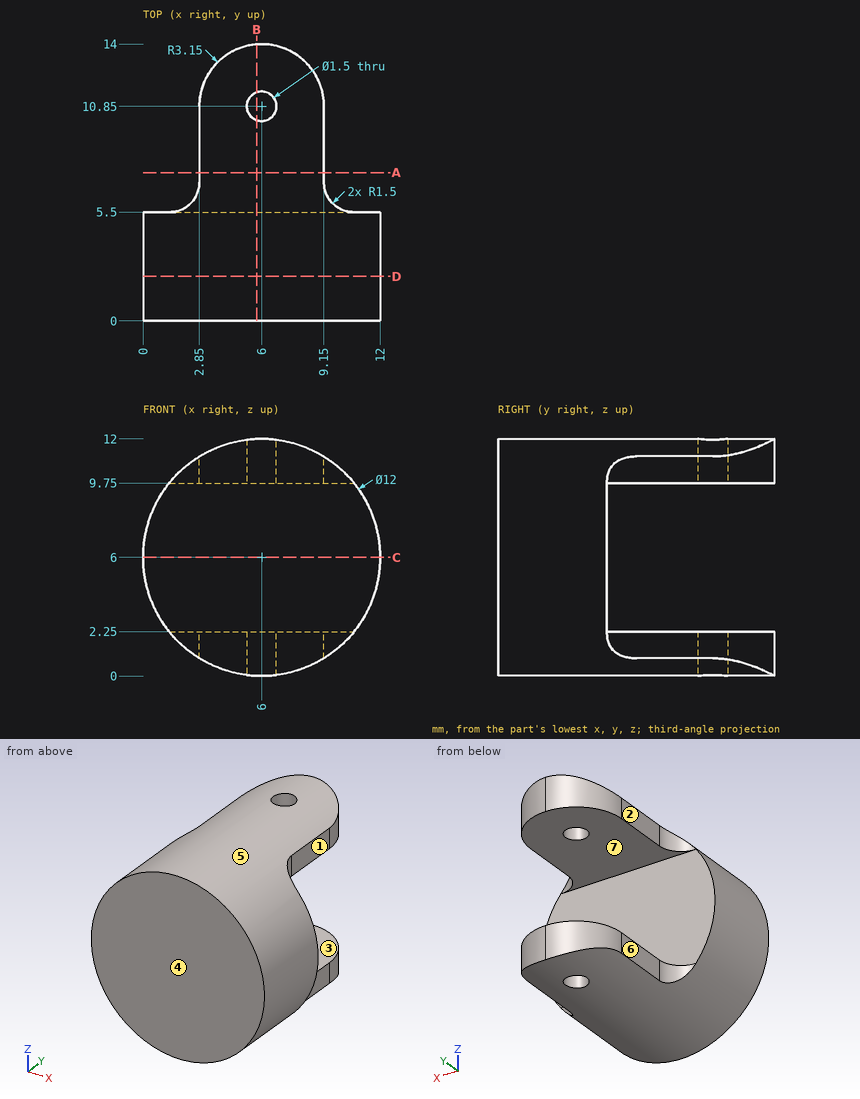
Design review of the part shown in the three views and the two pictorial views. Dimensions are in mm from the part's minimum x, y and z. A direction names the side the tool comes from. Round coordinates to 2 decimals unless told otherwise and drop trailing zeros. Loops run counter-clockwise (first coordinate to the right, second up) from the corner with the lowest first, then second, coordinate; pieces in that order, holes last. Notation, with made-up numbers: M 26.5,29.25 L 51.5,29.25 A23 ccw 51.5,48.25 Z; hole C -10,-13.5 d9. An arc over 180 degrees is marked long. Put each result on its own line as item: value.
Q1. Consider section A-A, the plane y = 7.5. Give the boundary of the cut face in (x, z), then the cut area to 3 significant figures.
Result set:
outline: M 2.85,0.89 A6 ccw 9.15,0.89 L 9.15,2.25 L 2.85,2.25 Z; M 2.85,9.75 L 9.15,9.75 L 9.15,11.11 A6 ccw 2.85,11.11 Z
area: 24.7 mm²
Q2. Consider section C-C, the plane z = 6. Give the boundary of the cut face in (x, y).
Result set:
outline: M 0,0 L 12,0 L 12,5.5 L 0,5.5 Z
Q3. Consider section B-B, the plane x = 5.75. Give the boundary of the cut face in (y, z).
Result set:
outline: M 0,0.01 L 10.14,0.01 L 10.14,2.25 L 5.5,2.25 L 5.5,9.75 L 10.14,9.75 L 10.14,11.99 L 0,11.99 Z; M 11.56,0.01 L 13.99,0.01 L 13.99,2.25 L 11.56,2.25 Z; M 11.56,9.75 L 13.99,9.75 L 13.99,11.99 L 11.56,11.99 Z
Q4. Mouldability with a two-part tool opening along Z and no side actions: class the marked faces 5, 6 and 7 as released by +Z, released by -Z, zero draft, split by the parting line, or undercut.
Result set:
face 5: split by the parting line
face 6: zero draft
face 7: undercut
Q5. Consider section D-D, the plane y = 2.25. Give the boundary of the cut face in (x, z).
Result set:
outline: C 6,6 d12
Q6. For pin 1 (1.5 mm diameter, centred on y = 8.5, z = 2, fed in from +X); pin 2 (0.7 mm diameter, centred on y = 9.5, z = 10.5, fed in from -X); pin 3 (6 mm diameter, centred on x = 2, y = 1.5, fed in from -Z), all flat-tipped, find the tip position at first contact; note any pin that passes through.
Result set:
pin 1: stops at x = 9.15
pin 2: stops at x = 2.85
pin 3: stops at z = 0.08
Q7. Machinability: for the marked faces 1, 2, 3 and 4, which of the approach directions +Z, -Z, +X, -X, +Y, -Y give a long, thin tool a straight path to every point of the face, cutting with its end or side? Answer none if there is none.
Result set:
face 1: +Z, -Z, +X, +Y
face 2: +Z, -Z, -X, +Y
face 3: +X, -X, +Y
face 4: +Z, -Z, +X, -X, -Y
Q8. To check wall thickness, follow L1, parallel to Z at x = 6.25, y = 8; L2, parallel to Y at x = 2.5, z = 7; L3, parallel to Z at x = 3.25, y = 9.25. State the ranges of each line that lie inside material, in increasing order.
Result set:
L1: z = 0.01 to 2.25, 9.75 to 11.99
L2: y = 0 to 5.5
L3: z = 0.67 to 2.25, 9.75 to 11.33
